from build123d import *

# Parameters (mm, degrees)
SKETCH1_R           = 1.75
SKETCH1_R_2         = 0.9
BOSS_EXTRUDE1_DEPTH = 2


with BuildPart() as part:
    # Sketch1 → Boss-Extrude1 (new body)
    with BuildSketch(Plane.XY):
        with BuildLine():
            ThreePointArc((1.50092417, 4.24231383), (-4.181288107, -1.663379022), (4.004901939, -2.052013757))
            ThreePointArc((4.004901939, -2.052013757), (4.731552678, -1.263858953), (5.760820585, -0.96416433))
            ThreePointArc((5.760820585, -0.96416433), (6.246121173, -0.970729914), (6.730453105, -1.002072336))
            ThreePointArc((6.730453105, -1.002072336), (7.628385483, -1.309353486), (8.28357181, -1.995964829))
            ThreePointArc((8.28357181, -1.995964829), (15.423311106, -1.583283146), (10.820810187, 3.890579172))
            ThreePointArc((10.820810187, 3.890579172), (9.607869973, 3.729173943), (8.387408257, 3.817201272))
            ThreePointArc((8.387408257, 3.817201272), (6.296455304, 4.03039557), (4.196647208, 3.939060928))
            ThreePointArc((4.196647208, 3.939060928), (2.831422573, 3.936340457), (1.50092417, 4.24231383))
        make_face()
        Circle(SKETCH1_R, mode=Mode.SUBTRACT)
        with Locations((11.75, 0)):
            Circle(SKETCH1_R_2, mode=Mode.SUBTRACT)
    extrude(amount=BOSS_EXTRUDE1_DEPTH)


solid = part.part
CAD build for the part. Positions are in the model's coordinates, mm. A direction names the side the tool comes from. Round coordinates to 2 decimals unless told otherwise and drop trailing zeros. Loops run counter-clockwise (first coordinate to the right, second up) from the corner with the lowest first, then second, coordinate; pieces in that order, holes last. Notation, with made-up numbers: (52, 32.25) - (72, 32.25) arc R23 ccw to (72, 45.25) - close; hole circle Ø8 at (-13.5, 31.25). An arc over 180 degrees is marked (long way). Put each result on its own line as item: value.
1. Slice it at A-A on x = 11.75. List the corners of the cut face in (y, z).
Geometry check:
outline: (-4, 0) - (-0.9, 0) - (-0.9, 2) - (-4, 2) - close; (0.9, 0) - (4, 0) - (4, 2) - (0.9, 2) - close
2. Pin check, flat tips, straight feed: P1, Ø1, axis at y = 2, z = 1, coming from the -X side; P2, Ø1.4, axis at x = 11.75, y = 0, coming from the -Z side. Stop position of each tip, or through.
Geometry check:
P1: x = -4.24
P2: through
3. Wall check: line 1 (Y direction, x = 11.75, z = 1.65); line 2 (Y direction, x = 0, z = 1.1); line 3 (X direction, y = 1.5, z = 0.45). Give the ranges that are in metal, low to high.
Geometry check:
line 1: -4 to -0.9, 0.9 to 4
line 2: -4.5 to -1.75, 1.75 to 4.5
line 3: -4.24 to -0.9, 0.9 to 15.46
4. Slice it at C-C on y = -3. List the corners of the cut face in (x, z), and give its area (3 significant figures).
Geometry check:
outline: (-3.35, 0) - (3.35, 0) - (3.35, 2) - (-3.35, 2) - close; (9.1, 0) - (14.4, 0) - (14.4, 2) - (9.1, 2) - close
area: 24.0 mm²
5. 3-axis set-ups, long thin cutter, end or side, ignore diameter. For faces 3 (the cylindrical face through (6.24, -0.97, 0.99)), 4 (the cylindrical face through (2.85, 3.934, 0.986)): which of +Z, -Z, +X, -X, +Y, -Y reach the whole face in a straight line?
Geometry check:
face 3: +Z, -Z, -Y
face 4: +Z, -Z, +Y
6. Two-plate mould, pull along X, no slides. Class faces 1 (the flat face through (5, 0, 0)), 2 (the cylindrical face through (6.33, 4.03, 0.99)): released by +X, released by -X, zero draft, split by the parting line, or undercut.
Geometry check:
face 1: zero draft
face 2: undercut
7. Slice it at B-B on y = 0. List the corners of the cut face in (x, z), and give its area (3 significant figures).
Geometry check:
outline: (-4.5, 0) - (-1.75, 0) - (-1.75, 2) - (-4.5, 2) - close; (1.75, 0) - (10.85, 0) - (10.85, 2) - (1.75, 2) - close; (12.65, 0) - (15.75, 0) - (15.75, 2) - (12.65, 2) - close
area: 29.9 mm²
8. Slice it at D-D on z = 1. List the corners of the cut face in (x, y) (3 decimals), and give its area (3 significant figures).
Geometry check:
outline: (1.501, 4.242) arc R4.5 ccw (long way) to (4.005, -2.052) arc R2 cw to (5.761, -0.964) arc R9.5 cw to (6.73, -1.002) arc R2 cw to (8.284, -1.996) arc R4 ccw (long way) to (10.821, 3.891) arc R6 cw to (8.387, 3.817) arc R14.5 ccw to (4.197, 3.939) arc R6 cw to start; hole circle Ø3.5 at (0, 0); hole circle Ø1.8 at (11.75, 0)
area: 124 mm²
